Autodesk Inventor part; units mm, degrees
ref_plane "Start Plane" through (0, 0, -10.9503) normal (0, 0, 1) x (1, 0, 0)
ref_plane "End Plane" through (0, 0, 80.417) normal (0, 0, 1) x (1, 0, 0)
ref_plane "Work Plane4" through (0, -10, 85) normal (0, 0.7071, 0.7071) x (1, 0, 0)
ref_plane "Start Plane" through (0, 0, -10.9503) normal (0, 0, 1) x (1, 0, 0)
ref_plane "End Plane" through (0, 0, 80.417) normal (0, 0, 1) x (1, 0, 0)
sketch "Sketch" plane through (0, 0, 0) normal (0, 0, 1) x (1, 0, 0)
  line L0 (-10, -7) -> (-10, 7)
  line L1 (-7, 10) -> (7, 10)
  line L2 (10, 7) -> (10, -7)
  line L3 (7, -10) -> (-7, -10)
  arc A0 (-10, -7) -> (-7, -10) centre (-7, -7) ccw
  arc A1 (-7, 10) -> (-10, 7) centre (-7, 7) ccw
  arc A2 (10, 7) -> (7, 10) centre (7, 7) ccw
  arc A3 (7, -10) -> (10, -7) centre (7, -7) ccw
  arc A4 (-7, 8) -> (-8, 7) centre (-7, 7) ccw
  line L4 (-7, 8) -> (7, 8)
  arc A5 (8, 7) -> (7, 8) centre (7, 7) ccw
  line L5 (8, 7) -> (8, -7)
  arc A6 (7, -8) -> (8, -7) centre (7, -7) ccw
  line L6 (7, -8) -> (-7, -8)
  arc A7 (-8, -7) -> (-7, -8) centre (-7, -7) ccw
  line L7 (-8, -7) -> (-8, 7)
  line L8 (0, 14.8698) -> (0, -14.8698) construction
  line L9 (-14.8698, 0) -> (14.8698, 0) construction
  dimension "d7" = 3
  dimension "d10" = 20
  dimension "d11" = 20
  dimension "d12" = 2
  dimension "d15" = 10
  dimension "d16" = 10
extrude "Body" add sketch "Sketch" along normal up to surface (91.3673 mm away) from surface at -10.9503
sketch "Sketch3" plane through (0, 0, 0) normal (0, 0, 1) x (1, 0, 0)
  line L0 (0, 0) -> (10, 0)
ref_plane "Work Plane3" through (0, 0, 0) normal (0, -1, 0) x (1, 0, 0)
sketch "Sketch4" plane through (0, 0, 0) normal (0, -1, 0) x (1, 0, 0)
  line L0 (-2, -10.9503) -> (12, -10.9503)
  line L1 (-2, 80.417) -> (12, 80.417)
  dimension "d18" = 91.3673
ref_plane "Work Plane4" through (0, -10, 85) normal (0, 0.7071, 0.7071) x (1, 0, 0)
split "Split1" plane through (0, -10, 85) removes the side toward (0, 0.7071, 0.7071)
ref_plane "Work Plane5" through (9.9561, -8.1221, -10) normal (-0.4759, 0.3882, -0.7892) x (-0.0742, 0.8764, 0.4759)
split "Split2" plane through (9.9561, -8.1221, -10) removes the side toward (-0.4759, 0.3882, -0.7892)
ref_plane "Work Plane6" through (10, 0, 80.417) normal (-0.4763, 0, 0.8793) x (0.8793, 0, 0.4763)
split "Split3" plane through (10, 0, 80.417) removes the side toward (-0.4763, 0, 0.8793)
equation "\"d7\" = G_IR"
equation "\"d10\" = G_H"
equation "\"d11\" = G_W"
equation "\"d12\" = G_T"
equation "\"d15\" = 0.5 * d10"
equation "\"d16\" = 0.5 * d11"
equation "\"d3\" = G_L"
equation "\"G_W\" = 20"
equation "\"G_H\" = 20"
equation "\"G_T\" = 2"
equation "\"G_IR\" = 3"
equation "\"G_L\" = 90.40511"
equation "\"G_OFFSET_START\" = 10.95031"
equation "\"G_OFFSET_END\" = 5.41698"
equation "\"d13\" = -G_OFFSET_START"
equation "\"d14\" = G_OFFSET_END + B_L"
equation "\"B_L\" = 75"
properties part number "ISO 12633-2 - 20x20x2 - 90.41" material "Steel, Mild"
Geometry: final body of the model. Coordinates: model frame, mm. A direction names the side the tool comes from. Coordinates: 2 decimals unless noted, no trailing zeros. Loops run counter-clockwise (first coordinate to the right, second up) from the corner with the lowest first, then second, coordinate; pieces in that order, holes last. Notation, with made-up numbers: M 57.5,75.5 L 77.5,75.5 A13 ccw 77.5,81.5 Z; hole C 23.5,20.5 d5. An arc over 180 degrees is marked long. One line per item, written item: value. Start each with the question number.
1) Cut plane B-B (y = -2). Return loops of the section in (x, z), then the cut area to 3 significant figures.
2) Cut plane A-A (z = 64). Return loops of the section in (x, y), then the cut area to 3 significant figures.
3) Cut plane D-D (z = 4). Return loops of the section in (x, y).
4) Reachability of faces 1 (the flat face through (3, 9, 66)), 2 (the flat face through (-8, 0, 36)) from +Z, -Z, +X, -X, +Y, -Y: full face, straight path, thin tool, end or side. Return the list, or none.
5) Pin query (flat end, axial travel): P1, Ø6, axis at x = -4, y = -2.5, coming from the -Z side. Return the tip coordinate at first contact, or that it passes through.
6) Draft query along Y for faces 3 (the cylindrical face through (9.1, 9.14, 32.21)), 4 (the flat face through (0, -8, 35)), 5 (the flat face through (10, 0, 35)). Return one class per face: released by +Y, released by -Y, zero draft, split by the parting line, or undercut.
7) Material intervals for L1, parallel to X at y = 4, z = 37.5; L2, parallel to X at y = -6.25, z = 1, sorted ascending. Write a range as from..to.
8) Cut plane C-C (x = 1). Return loops of the section in (y, z), then the cut area to 4 significant figures.
Evaluation:
1. outline: M -10,5.05 L -8,3.84 L -8,70.67 L -10,69.58 Z; M 8,-5.81 L 10,-7.02 L 10,77 L 8,77 Z
1. area: 298 mm^2
2. outline: M -10,-7 A3 ccw -7,-10 L 7,-10 A3 ccw 10,-7 L 10,7 A3 ccw 7,10 L -7,10 A3 ccw -10,7 Z; hole M -8,-7 A1 ccw -7,-8 L 7,-8 A1 ccw 8,-7 L 8,7 A1 ccw 7,8 L -7,8 A1 ccw -8,7 Z
2. area: 137 mm^2
3. outline: M -10,-7 A3 ccw -7,-10 L 7,-10 A3 ccw 10,-7 L 10,7 A3 ccw 7,10 L 1.52,10 L -0.11,8 L 7,8 A1 cw 8,7 L 8,-7 A1 cw 7,-8 L -7,-8 A1 cw -8,-7 L -8,-1.67 L -10,-4.12 Z
4. face 1: +Z, +X, -X, +Y
4. face 2: +Z, -Z
5. P1: through
6. face 3: released by +Y
6. face 4: undercut
6. face 5: zero draft
7. L1: -10..-8, 8..10
7. L2: 8..10
8. outline: M -10,-5.52 L -8,-4.54 L -8,75.54 L -10,75.54 Z; M 8,3.33 L 10,4.31 L 10,65 L 8,67 Z
8. area: 285.5 mm^2
